from build123d import *

# Parameters (mm, degrees)
SKETCH1_W               = 44.45
SKETCH1_H               = 44.45
SKETCH1_W_2             = 38.1
SKETCH1_H_2             = 38.1
BOSS_EXTRUDE1_DEPTH     = 844.55
F_1_4_CLEARANCE_HOLE1_D = 7.14248


with BuildPart() as part:
    # Sketch1 → Boss-Extrude1 (new body)
    with BuildSketch(Plane(origin=(0, 0, 0), x_dir=(1, 0, 0), z_dir=(0, 1, 0))):
        Rectangle(SKETCH1_W, SKETCH1_H)
        Rectangle(SKETCH1_W_2, SKETCH1_H_2, mode=Mode.SUBTRACT)
    extrude(amount=BOSS_EXTRUDE1_DEPTH)

    # 1/4 Clearance Hole1 (through all)
    with Locations(Plane.ZY.offset(22.225)):
        with Locations((0, 803.275), (0, 41.275), (0, 822.721875), (0, 21.828125)):
            Hole(F_1_4_CLEARANCE_HOLE1_D / 2)


solid = part.part
The model under review builds one solid part; all positions refer to its coordinate system, in mm. A direction names the side the tool comes from. Give positions to 0.01 mm unless a question says otherwise; leave off trailing zeros. Write each loop counter-clockwise with the first axis right and the second up, starting at its lowest first coordinate (ties: lowest second). Pieces come first, ordered by that corner, then holes. Notation, with made-up numbers: M -20,2.5 L 8,2.5 A21 ccw 8,23.5 Z; hole C 10.25,31.25 d6. An arc over 180 degrees is marked long. One line per question, with ' | ' between items. Start each with the question number.
Item 1: Draft analysis for pull direction Z (two halves, no side actions). For faces 3 (the flat face through (-22.225, 416, 0)), 4 (the flat face through (0, 416, -19.05)), 5 (the flat face through (0, 416, 22.225)), state which applies: released by +Z, released by -Z, zero draft, split by the parting line, or undercut.
Item 2: We need section A-A on y = 531. Write out the cut boundary in (x, z) (3 decimals).
Item 3: Wall thickness on line 1 (Y direction, x = -20, z = 0); line 2 (Z direction, x = 9, y = 607) (3 decimals): over which ranges is each line inside the solid? List them lowest first. Write a range as from..to.
Item 4: For pin 1 (8 mm diameter, centred on y = 822.72, z = 0, fed in from -X) (3 decimals); pin 2 (12 mm diameter, centred on x = 12, z = 13, fed in from -Y), all flat-tipped, find the tip position at first contact; note any pin that passes through.
Item 5: For faces 1 (the flat face through (-19.05, 416, 0)), 2 (the flat face through (19.4, 0, -0.3)), list the 3-axis set-ups (+Z, -Z, +X, -X, +Y, -Y) from which the entire face can be reached by the end or side of a thin tool; tool diameter is ignored.
Item 6: We need section B-B on x = 8.5. Write out the cut boundary in (y, z) (3 decimals), plus the area to 3 significant figures.
Results found:
1) face 3: zero draft | face 4: undercut | face 5: released by +Z
2) outline: M -22.225,-22.225 L 22.225,-22.225 L 22.225,22.225 L -22.225,22.225 Z; hole M -19.05,-19.05 L 19.05,-19.05 L 19.05,19.05 L -19.05,19.05 Z
3) line 1: y = 0..18.26, 25.4..37.7, 44.85..799.7, 806.85..819.15, 826.29..844.55 | line 2: z = -22.225..-19.05, 19.05..22.225
4) pin 1: stops at x = -22.225 | pin 2: passes through
5) face 1: +Y, -Y | face 2: +Z, -Z, +X, -X, -Y
6) outline: M 0,-22.225 L 844.55,-22.225 L 844.55,-19.05 L 0,-19.05 Z; M 0,19.05 L 844.55,19.05 L 844.55,22.225 L 0,22.225 Z | area: 5,360 mm2
